```python
from build123d import *

# Parameters (mm, degrees)
F2_R     = 11
F3_DEPTH = 25
F4_R     = 20
F5_DEPTH = 25


with BuildPart() as f1:
    # F0 (on Front) → F1 (revolve)
    with BuildSketch(Plane.XZ):
        with BuildLine():
            Line((0, 25), (0, -25))
            ThreePointArc((0, -25), (25, 0), (0, 25))
        make_face()
    revolve(axis=Axis((0, 0, 0), (0, 0, -1)))

    # F2 (on Front) → F3 (cut, symmetric)
    with BuildSketch(Plane.XZ):
        with Locations((16, 0)):
            Circle(F2_R)
    extrude(amount=F3_DEPTH, both=True, mode=Mode.SUBTRACT)

    # F4 (on Front) → F5 (cut, symmetric)
    with BuildSketch(Plane.XZ):
        with Locations((-20, 0)):
            Circle(F4_R)
    extrude(amount=F5_DEPTH, both=True, mode=Mode.SUBTRACT)


solid = f1.part
```
CAD build for the part. Positions are in the model's coordinates, mm. Give positions to 0.01 mm unless a question says otherwise; leave off trailing zeros. Write each loop counter-clockwise with the first axis right and the second up, starting at its lowest first coordinate (ties: lowest second). Pieces come first, ordered by that corner, then holes. Notation, with made-up numbers: M -37.5,-1.75 L 13.5,-1.75 A29 ccw 13.5,31.25 Z; hole C -24.5,25.25 d6. An arc over 180 degrees is marked long. Return JSON: item names as keys, results as strings. Group by question number.
(1) Band-saw the part on D-D (x = 17). Give the cut face in (y, z).
(2) Band-saw the part on B-B (z = 12.5). Give the cut face in (x, y), and give its area (3 significant figures).
(3) Flat gauge pins, fed straight in: pin 1 Ø1 at (y, z) = (15, 11.5) entering from +X; pin 2 Ø2 at (x, y) = (-4.5, -8) entering from +Z; pin 3 Ø10 at (x, z) = (17.5, -13) entering from +Y. Where does each tip first touch, or does it go through?
(4) Band-saw the part on C-C (y = 18.5). Give the cut face in (x, z).
(5) Band-saw the part on A-A (x = -9). Give the cut face in (y, z), and give its area (3 significant figures).
(6) Drill centre lines: L1, parallel to Z at x = -2.5, y = -13; L2, parallel to X at y = -9.5, z = 0; L3, parallel to Z at x = 16, y = 10. Where is each one in solid material? Low to high. Write a range as [from, to].
Entries:
{
 "1": {"outline": "M -14.7,-10.95 A18.33 ccw 14.7,-10.95 Z; M -14.7,10.95 L 14.7,10.95 A18.33 ccw Z"},
 "2": {"outline": "M -4.39,-21.2 A21.65 ccw long -4.39,21.2 Z", "area": "925 mm^2"},
 "3": {"pin 1": "stops at x = 16.92", "pin 2": "stops at z = 23.62", "pin 3": "stops at y = 18.45"},
 "4": {"outline": "M -7.07,-15.26 A16.82 ccw 13.05,-10.6 A11 cw 13.05,10.6 A16.82 ccw -7.07,15.26 A20 cw Z"},
 "5": {"outline": "M -16.28,-16.7 A23.32 ccw 16.28,-16.7 Z; M -16.28,16.7 L 16.28,16.7 A23.32 ccw Z", "area": "297 mm^2"},
 "6": {"L1": "z = [-21.21, -9.68], [9.68, 21.21]", "L2": "x = [0, 5]", "L3": "z = [-16.4, -11], [11, 16.4]"}
}
